from build123d import *

# Parameters (mm, degrees)
EXTRUDE_1_DEPTH      = 7.56
EXTRUDE_1_DEPTH_BACK = 7.56
SKETCH_1_R           = 25
SKETCH_1_R_2         = 4
SKETCH_4_R           = 2.1
CUT_EXTRUDE_1_DEPTH  = 37.15457924
SKETCH_5_R           = 2.1
CUT_EXTRUDE_2_DEPTH  = 37.154579261
CHAMFER_1_SIZE       = 0.5


with BuildPart() as part:
    # Sketch 1 → Extrude 1 (new, two sides: drawn at the far end of the back side and taken through both)
    with BuildSketch(Plane.XY.offset(-EXTRUDE_1_DEPTH_BACK)):
        Circle(SKETCH_1_R)
        Circle(SKETCH_1_R_2, mode=Mode.SUBTRACT)
    extrude(amount=EXTRUDE_1_DEPTH + EXTRUDE_1_DEPTH_BACK)

    # Sketch 3 → Cut-Revolve 2 (revolve, cut)
    with BuildSketch(Plane(origin=(0, 0, 0), x_dir=(0, 0, -1), z_dir=(1, 0, 0)), mode=Mode.PRIVATE) as cut_revolve_2_sk:
        Polygon((-5, 25), (5, 25), (2.5, 16.5), (-2.5, 16.5), align=None)
    revolve(cut_revolve_2_sk.sketch.rotate(Axis((0, 0, 7.56), (0, 0, -1)), 90), axis=Axis((0, 0, 7.56), (0, 0, -1)), mode=Mode.SUBTRACT)

    # Sketch 4 → Cut-Extrude 1 (cut, through all)
    with BuildSketch(Plane(origin=(0, 0, 0), x_dir=(1, 0, 0), z_dir=(0, 1, 0))):
        with Locations(Location((0, 0, 0), (0, 0, 90))):
            Circle(SKETCH_4_R)
    extrude(amount=CUT_EXTRUDE_1_DEPTH, mode=Mode.SUBTRACT)

    # Sketch 5 → Cut-Extrude 2 (cut, through all)
    with BuildSketch(Plane(origin=(0, 0, 0), x_dir=(0, 0, -1), z_dir=(1, 0, 0))):
        with Locations(Location((0, 0, 0), (0, 0, 180))):
            Circle(SKETCH_5_R)
    extrude(amount=CUT_EXTRUDE_2_DEPTH, mode=Mode.SUBTRACT)

    # Chamfer 1
    chamfer_1_edges = [part.edges().sort_by_distance(p)[0] for p in [
        (-25, 0, -7.56),
        (-4, 0, -7.56),
        (-25, 0, 7.56),
        (-4, 0, 7.56),
    ]]
    chamfer(chamfer_1_edges, length=CHAMFER_1_SIZE)


solid = part.part
Input: part model. Units: mm. Frame: model coordinates. A direction names the side the tool comes from. Give positions to 0.01 mm unless a question says otherwise; leave off trailing zeros. Write each loop counter-clockwise with the first axis right and the second up, starting at its lowest first coordinate (ties: lowest second). Pieces come first, ordered by that corner, then holes. Notation, with made-up numbers: M 88.25,-2 L 136.25,-2 A22 cw 136.25,35 Z; hole C 14.25,-19 d11. An arc over 180 degrees is marked long. Write item = value, one per line. Start each with the question number.
1) Cut plane D-D on z = 3.75. Return the cut outline in (x, y), then the cut area to 3 significant figures.
2) Cut plane A-A on y = 0. Return the cut outline in (x, z), then the cut area to 3 significant figures.
3) Cut plane C-C on z = 0. Return the cut outline in (x, y).
4) First-contact query: pin 1 Ø3.5 at (y, z) = (0, 0) entering from +X; pin 2 Ø3 at (x, y) = (-16, -20) entering from -Z; pin 3 Ø1.5 at (x, z) = (-14, -0.5) entering from -Y; pin 4 Ø3 at (y, z) = (10, -6) entering from -X. Flat tips, straight axial feed; report the tip coordinate or a pass-through.
5) Reachability of faces 1 (the conical face through (16.13, -5.08, -2.62)), 2 (the cylindrical face through (23.846, 7.509, 6.016)), 3 (the cylindrical face through (-0.631, 9.862, -2.003)), 4 (the cylindrical face through (9.861, -0.631, 2.003)) from +Z, -Z, +X, -X, +Y, -Y: full face, straight path, thin tool, end or side. Return the list, or none.
6) Draft query along X for faces 5 (the cylindrical face through (-3.2, -2.4, -0.1)), 6 (the flat face through (5, 0, -7.56)), 7 (the conical face through (-2.217, -16.887, 2.656)). Return one class per face: +X half, -X half, draft (parallel to the pull), parting line (faces both ways), or undercut.
7) Material intervals for line 1 along Z through (x, y) = (20, -2); line 2 along Z through (x, y) = (1, 17.5); line 3 along Y through (x, z) = (8, 0), sorted ascending. Write a range as [from, to].
Solved:
q1.outline = C 0,0 d41.5; hole C 0,0 d8
q1.area = 1,300 mm2
q2.outline = M -25,-7.06 L -24.5,-7.56 L -4.5,-7.56 L -4,-7.06 L -4,7.06 L -4.5,7.56 L -24.5,7.56 L -25,7.06 L -25,5 L -16.5,2.5 L -16.5,-2.5 L -25,-5 Z; M 4,-7.06 L 4.5,-7.56 L 24.5,-7.56 L 25,-7.06 L 25,-5 L 16.5,-2.5 L 16.5,-2.1 L 4,-2.1 Z; M 4,2.1 L 16.5,2.1 L 16.5,2.5 L 25,5 L 25,7.06 L 24.5,7.56 L 4.5,7.56 L 4,7.06 Z
q2.area = 454 mm2
q3.outline = M -2.1,3.4 L -2.1,16.37 A16.5 ccw long 16.37,-2.1 L 3.4,-2.1 A4 cw long Z; M 2.1,3.4 A4 cw 3.4,2.1 L 16.37,2.1 A16.5 ccw 2.1,16.37 Z
q4.pin_1 = -3.6
q4.pin_2 = -7.56
q4.pin_3 = -9.83
q4.pin_4 = -23.51
q5.face_1 = none
q5.face_2 = +Z, -Z
q5.face_3 = +Y
q5.face_4 = +X
q6.face_5 = undercut
q6.face_6 = draft
q6.face_7 = parting line
q7.line_1 = [-7.56, -3.56], [3.56, 7.56]
q7.line_2 = [-7.56, -2.8], [2.8, 7.56]
q7.line_3 = [-14.43, -2.1], [2.1, 14.43]
